Build history of the part. All positions in model axes, mm. A direction names the side the tool comes from. Round coordinates to 2 decimals unless told otherwise and drop trailing zeros. Write each loop counter-clockwise with the first axis right and the second up, starting at its lowest first coordinate (ties: lowest second). Pieces come first, ordered by that corner, then holes. Notation, with made-up numbers: M -36,77.5 L -24,77.5 A21 cw -24,97.5 Z; hole C -19.5,-40 d1. An arc over 180 degrees is marked long. One line per item, written item: value. Start each with the question number.
```python
from build123d import *

# Parameters (mm, degrees)
F0_R      = 30
F1_DEPTH  = 10
F2_R      = 30
F2_R_2    = 27.5
F3_DEPTH  = 40
F5_DEPTH  = 35
F6_DEPTH  = 35
F7_DEPTH  = 0.001
F8_ANGLE  = 90
F10_DEPTH = 100


with BuildPart() as f1:
    # F0 (on Top) → F1 (new body)
    with BuildSketch(Plane.XY):
        Circle(F0_R)
    extrude(amount=F1_DEPTH)

    # F2 (on face) → F3 (join)
    with BuildSketch(Plane.XY.offset(10)):
        Circle(F2_R)
        Circle(F2_R_2, mode=Mode.SUBTRACT)
    extrude(amount=F3_DEPTH)

    # F4 (on Front) → F5 (cut)
    with BuildSketch(Plane.XZ):
        with BuildLine():
            ThreePointArc((-1.0021791073, 29.8523980864), (-1.0005448065, 29.9261910009), (-1, 30))
            ThreePointArc((-1, 30), (-7.2972686774, 34.8287776899), (-10.3268375915, 27.4943111812))
            Line((-10.3268375915, 27.4943111812), (-1.0021791073, 29.8523980864))
        make_face()
        with BuildLine():
            Line((-1.0021791073, 29.8523980864), (-10.3268375915, 27.4943111812))
            ThreePointArc((-10.3268375915, 27.4943111812), (-4.7741541244, 25.1525984394), (-1.0021791073, 29.8523980864))
        make_face()
        with BuildLine():
            ThreePointArc((-1.0021791073, 29.8523980864), (-4.7741541244, 25.1525984394), (-10.3268375915, 27.4943111812))
            Line((-10.3268375915, 27.4943111812), (-1.0021791073, 11.3924382934))
            Line((-1.0021791073, 11.3924382934), (-1.0021791073, 29.8523980864))
        make_face()
        with BuildLine():
            ThreePointArc((10.3268375915, 27.4943111812), (10.8287776899, 28.7027313226), (11, 30))
            ThreePointArc((11, 30), (5.9261910009, 34.9994551935), (1.0021791073, 29.8523980864))
            Line((1.0021791073, 29.8523980864), (10.3268375915, 27.4943111812))
        make_face()
        with BuildLine():
            Line((10.3268375915, 27.4943111812), (1.0021791073, 29.8523980864))
            ThreePointArc((1.0021791073, 29.8523980864), (4.7741541244, 25.1525984394), (10.3268375915, 27.4943111812))
        make_face()
        with BuildLine():
            ThreePointArc((10.3268375915, 27.4943111812), (4.7741541244, 25.1525984394), (1.0021791073, 29.8523980864))
            Line((1.0021791073, 29.8523980864), (1.0021791073, 11.3924382934))
            Line((1.0021791073, 11.3924382934), (10.3268375915, 27.4943111812))
        make_face()
    extrude(amount=-F5_DEPTH, mode=Mode.SUBTRACT)

    # F4 (on Front) → F6 (cut)
    with BuildSketch(Plane.XZ):
        with BuildLine():
            ThreePointArc((10.3268375915, 27.4943111812), (10.8287776899, 28.7027313226), (11, 30))
            ThreePointArc((11, 30), (5.9261910009, 34.9994551935), (1.0021791073, 29.8523980864))
            Line((1.0021791073, 29.8523980864), (10.3268375915, 27.4943111812))
        make_face()
        with BuildLine():
            Line((10.3268375915, 27.4943111812), (1.0021791073, 29.8523980864))
            ThreePointArc((1.0021791073, 29.8523980864), (4.7741541244, 25.1525984394), (10.3268375915, 27.4943111812))
        make_face()
        with BuildLine():
            ThreePointArc((10.3268375915, 27.4943111812), (4.7741541244, 25.1525984394), (1.0021791073, 29.8523980864))
            Line((1.0021791073, 29.8523980864), (1.0021791073, 11.3924382934))
            Line((1.0021791073, 11.3924382934), (10.3268375915, 27.4943111812))
        make_face()
        with BuildLine():
            ThreePointArc((-1.0021791073, 29.8523980864), (-1.0005448065, 29.9261910009), (-1, 30))
            ThreePointArc((-1, 30), (-7.2972686774, 34.8287776899), (-10.3268375915, 27.4943111812))
            Line((-10.3268375915, 27.4943111812), (-1.0021791073, 29.8523980864))
        make_face()
        with BuildLine():
            Line((-1.0021791073, 29.8523980864), (-10.3268375915, 27.4943111812))
            ThreePointArc((-10.3268375915, 27.4943111812), (-4.7741541244, 25.1525984394), (-1.0021791073, 29.8523980864))
        make_face()
        with BuildLine():
            ThreePointArc((-1.0021791073, 29.8523980864), (-4.7741541244, 25.1525984394), (-10.3268375915, 27.4943111812))
            Line((-10.3268375915, 27.4943111812), (-1.0021791073, 11.3924382934))
            Line((-1.0021791073, 11.3924382934), (-1.0021791073, 29.8523980864))
        make_face()
    extrude(amount=F6_DEPTH, mode=Mode.SUBTRACT)


with BuildPart() as f7:
    # F4 (on Front) → F7 (new body)
    with BuildSketch(Plane.XZ):
        with BuildLine():
            ThreePointArc((10.3268375915, 27.4943111812), (10.8287776899, 28.7027313226), (11, 30))
            ThreePointArc((11, 30), (5.9261910009, 34.9994551935), (1.0021791073, 29.8523980864))
            Line((1.0021791073, 29.8523980864), (10.3268375915, 27.4943111812))
        make_face()
        with BuildLine():
            Line((10.3268375915, 27.4943111812), (1.0021791073, 29.8523980864))
            ThreePointArc((1.0021791073, 29.8523980864), (4.7741541244, 25.1525984394), (10.3268375915, 27.4943111812))
        make_face()
        with BuildLine():
            ThreePointArc((10.3268375915, 27.4943111812), (4.7741541244, 25.1525984394), (1.0021791073, 29.8523980864))
            Line((1.0021791073, 29.8523980864), (1.0021791073, 11.3924382934))
            Line((1.0021791073, 11.3924382934), (10.3268375915, 27.4943111812))
        make_face()
    extrude(amount=F7_DEPTH)


with BuildPart() as f7b:
    # F4 (on Front) → F7, piece 2 (new body)
    with BuildSketch(Plane.XZ):
        with BuildLine():
            ThreePointArc((-1.0021791073, 29.8523980864), (-1.0005448065, 29.9261910009), (-1, 30))
            ThreePointArc((-1, 30), (-7.2972686774, 34.8287776899), (-10.3268375915, 27.4943111812))
            Line((-10.3268375915, 27.4943111812), (-1.0021791073, 29.8523980864))
        make_face()
        with BuildLine():
            Line((-1.0021791073, 29.8523980864), (-10.3268375915, 27.4943111812))
            ThreePointArc((-10.3268375915, 27.4943111812), (-4.7741541244, 25.1525984394), (-1.0021791073, 29.8523980864))
        make_face()
        with BuildLine():
            ThreePointArc((-1.0021791073, 29.8523980864), (-4.7741541244, 25.1525984394), (-10.3268375915, 27.4943111812))
            Line((-10.3268375915, 27.4943111812), (-1.0021791073, 11.3924382934))
            Line((-1.0021791073, 11.3924382934), (-1.0021791073, 29.8523980864))
        make_face()
    extrude(amount=F7_DEPTH)


with BuildPart() as f7b_1:
    # F8: moved
    add(f7b.part.rotate(Axis((0, 0, 0), (0, 0, -1)), F8_ANGLE))


with BuildPart() as f7_1:
    # F8: moved
    add(f7.part.rotate(Axis((0, 0, 0), (0, 0, -1)), F8_ANGLE))


with BuildPart() as f7_2:
    # F9: moved
    add(f7_1.part.moved(Location((48.6, 0, 0))))


with BuildPart() as f7b_2:
    # F9: moved
    add(f7b_1.part.moved(Location((48.6, 0, 0))))


with BuildPart() as f10_tool:
    # F7_face (on face) → F10 (new body)
    with BuildSketch(Plane(origin=(48.6, -4.9596337945, 26.1247931076), x_dir=(0, 1, 0), z_dir=(1, 0, 0))):
        with BuildLine():
            Line((3.9574546871, -14.7323548142), (3.9574546871, 3.7276049788))
            ThreePointArc((3.9574546871, 3.7276049788), (-2.2662120811, 8.722608453), (-5.367203797, 1.3695180736))
            Line((-5.367203797, 1.3695180736), (3.9574546871, -14.7323548142))
        make_face()
        with BuildLine():
            Line((5.9618129018, -14.7323548142), (15.2864713859, 1.3695180736))
            ThreePointArc((15.2864713859, 1.3695180736), (12.18547967, 8.722608453), (5.9618129018, 3.7276049788))
            Line((5.9618129018, 3.7276049788), (5.9618129018, -14.7323548142))
        make_face()
    extrude(amount=-F10_DEPTH)


with BuildPart() as f1_1:
    add(f1.part)

    # F10: cut by f10_tool
    add(f10_tool.part, mode=Mode.SUBTRACT)


with BuildPart() as f7_3:
    add(f7_2.part)

    # F10: cut by f10_tool
    add(f10_tool.part, mode=Mode.SUBTRACT)


with BuildPart() as f7b_3:
    add(f7b_2.part)

    # F10: cut by f10_tool
    add(f10_tool.part, mode=Mode.SUBTRACT)


solid = f1_1.part
```
Item 1: Cut at B-B, the plane z = 24. Count the separate pieces of the cut face and the enclosed holes in it, plus the area to 3 significant figures.
Item 2: Which spindle directions (+Z, -Z, +X, -X, +Y, -Y) get a long thin tool onto all of the face, cutting with end or side? Do faces 5 (the flat face through (-1.002, 29, 20)), 6 (the flat face through (13.2, -24.3, 50)), 7 (the flat face through (29, 1.002, 21)). Say none if no direction does.
Item 3: Drill centre lines: line 1 (Y direction, x = 0, z = 28.5); line 2 (Y direction, x = 29, z = 30); line 3 (Z direction, x = -11.5, y = -18). Where is each one in solid material? Low to high.
Item 4: Cut at A-A, the plane x = 0. Write the cut outline in (y, z).
Item 5: Drop flat-ended pins along their axis: pin 1 (10 mm diameter, centred on x = 11, z = 21.5, fed in from +Y); pin 2 (12 mm diameter, centred on y = -8, z = 30, fed in from -X); pin 3 (10 mm diameter, centred on y = -20, z = 29.5, fed in from +X); pin 4 (8 mm diameter, centred on x = -6, z = 30, fed in from -Y). Give the stop position or say it passes through.
Item 6: Cut at D-D, the plane z = 44.5. Write the cut outline in (x, y).
Item 7: Two-plate mould, pull along X, no slides. Class faces 1 (the flat face through (0, 0, 0)), 2 (the cylindrical face through (12.69, -24.397, 29.72)), 3 (the flat face through (5.6, -28.2, 19.33)), 4 (the cylindrical face through (27.712, -11.49, 24.65)): pulls with the +X half, pulls with the -X half, needs draft (parallel to the pull), parting line crosses it, or undercut.
Computed values:
1. separate pieces: 8
1. enclosed holes: 0
1. area: 303 mm2
2. face 5: +Y, -Y
2. face 6: +Z, +X, -X, +Y, -Y
2. face 7: +X, -X
3. line 1: y = -30 to -27.5, 27.5 to 30
3. line 2: y = -1 to 1
3. line 3: z = 0 to 10
4. outline: M -30,0 L 30,0 L 30,50 L 27.5,50 L 27.5,10 L -27.5,10 L -27.5,50 L -30,50 Z
5. pin 1: stops at y = 29.36
5. pin 2: stops at x = -29.7
5. pin 3: stops at x = 25.98
5. pin 4: passes through
6. outline: C 0,0 d60; hole C 0,0 d55
7. face 1: needs draft
7. face 2: undercut
7. face 3: undercut
7. face 4: parting line crosses it
